Input: part model. Units: mm. Frame: model coordinates. A direction names the side the tool comes from. Coordinates: 2 decimals unless noted, no trailing zeros. Order: outer loops, then holes, each group sorted by start corner. A loop starts at its lowest first (then second) coordinate and runs counter-clockwise, first axis right, second up. Notation, with made-up numbers: M 50.25,-14 L 91.25,-14 A20 cw 91.25,17 Z; hole C 18.5,-23.75 d4. An arc over 180 degrees is marked long. Answer in a Markdown table with one row per item.
from build123d import *

# Parameters (mm, degrees)
ESQUISSE1_W             = 90
ESQUISSE1_H             = 65
ESQUISSE1_R             = 7
ESQUISSE1_R_2           = 13
BOSS_EXTRU_1_DEPTH      = 8
ESQUISSE2_R             = 13
BOSS_EXTRU_2_DEPTH      = 3
ESQUISSE3_R             = 7
ESQUISSE3_R_2           = 1.5
ENL_V_MAT_EXTRU_1_DEPTH = 4
ESQUISSE4_R             = 8
ENL_V_MAT_EXTRU_2_DEPTH = 5.5
ESQUISSE5_W             = 45
ESQUISSE5_H             = 8
ENL_V_MAT_EXTRU_3_DEPTH = 9
ESQUISSE6_R             = 1.65
ENL_V_MAT_EXTRU_4_DEPTH = 10
ESQUISSE7_R             = 1.65
ENL_V_MAT_EXTRU_5_DEPTH = 10


with BuildPart() as part:
    # Esquisse1 → Boss.-Extru.1 (new body)
    with BuildSketch(Plane.XY):
        with Locations((45, 32.5)):
            Rectangle(ESQUISSE1_W, ESQUISSE1_H)
        with Locations((70, 20)):
            Circle(ESQUISSE1_R, mode=Mode.SUBTRACT)
        with Locations((17, 20)):
            Circle(ESQUISSE1_R_2, mode=Mode.SUBTRACT)
        with Locations((25, 48)):
            Circle(ESQUISSE1_R_2, mode=Mode.SUBTRACT)
    extrude(amount=BOSS_EXTRU_1_DEPTH)

    # Esquisse2 → Boss.-Extru.2 (add)
    with BuildSketch(Plane(origin=(0, 0, 0), x_dir=(-1, 0, 0), z_dir=(0, 0, -1))):
        with Locations((-17, 20)):
            Circle(ESQUISSE2_R)
    extrude(amount=-BOSS_EXTRU_2_DEPTH)

    # Esquisse3 → Enlèv. mat.-Extru.1 (cut, through all)
    with BuildSketch(Plane.XY.offset(3)):
        with Locations((17, 20)):
            Circle(ESQUISSE3_R)
        with Locations((27, 20)):
            Circle(ESQUISSE3_R_2)
        with Locations((17, 10)):
            Circle(ESQUISSE3_R_2)
        with Locations((7, 20)):
            Circle(ESQUISSE3_R_2)
        with Locations((17, 30)):
            Circle(ESQUISSE3_R_2)
    extrude(amount=-ENL_V_MAT_EXTRU_1_DEPTH, mode=Mode.SUBTRACT)

    # Esquisse4 → Enlèv. mat.-Extru.2 (cut)
    with BuildSketch(Plane.XY.offset(8)):
        with Locations((70, 20)):
            Circle(ESQUISSE4_R)
    extrude(amount=-ENL_V_MAT_EXTRU_2_DEPTH, mode=Mode.SUBTRACT)

    # Esquisse5 → Enlèv. mat.-Extru.3 (cut, through all)
    with BuildSketch(Plane.XY.offset(8)):
        with Locations((67.5, 61)):
            Rectangle(ESQUISSE5_W, ESQUISSE5_H)
    extrude(amount=-ENL_V_MAT_EXTRU_3_DEPTH, mode=Mode.SUBTRACT)

    # Esquisse6 → Enlèv. mat.-Extru.4 (cut)
    with BuildSketch(Plane.ZY):
        with Locations((4, 7)):
            Circle(ESQUISSE6_R)
        with Locations((4, 45)):
            Circle(ESQUISSE6_R)
    extrude(amount=-ENL_V_MAT_EXTRU_4_DEPTH, mode=Mode.SUBTRACT)

    # Esquisse7 → Enlèv. mat.-Extru.5 (cut)
    with BuildSketch(Plane(origin=(0, 57, 0), x_dir=(1, 0, 0), z_dir=(0, 1, 0))):
        with Locations((85, -4)):
            Circle(ESQUISSE7_R)
        with Locations((55, -4)):
            Circle(ESQUISSE7_R)
    extrude(amount=-ENL_V_MAT_EXTRU_5_DEPTH, mode=Mode.SUBTRACT)


solid = part.part
1) Reachability of faces 1 (the face through (53.35, 52.07, 3.93)), 2 (the face through (10, 7, 4)), 3 (the face through (11, 14, 3)) from +Z, -Z, +X, -X, +Y, -Y: full face, straight path, thin tool, end or side. Return the list, or none.
Resolved:
| item | result |
|---|---|
| face 1 | +Y |
| face 2 | -X |
| face 3 | +Z |
2) Cut plane C-C, the plane x = 55. Output: boundary loops of the cut face in (y, z), and give its area (3 significant figures).
Resolved:
| item | result |
|---|---|
| outline | M 0,0 L 57,0 L 57,2.35 L 47,2.35 L 47,5.65 L 57,5.65 L 57,8 L 0,8 Z |
| area | 423 mm2 |
3) Cut plane B-B, the plane z = 4. Output: boundary loops of the cut face in (x, y), and give its area (3 significant figures).
Resolved:
| item | result |
|---|---|
| outline | M 0,0 L 90,0 L 90,57 L 86.65,57 L 86.65,47 L 83.35,47 L 83.35,57 L 56.65,57 L 56.65,47 L 53.35,47 L 53.35,57 L 45,57 L 45,65 L 0,65 L 0,46.65 L 10,46.65 L 10,43.35 L 0,43.35 L 0,8.65 L 10,8.65 L 10,5.35 L 0,5.35 Z; hole C 17,20 d26; hole C 25,48 d26; hole C 70,20 d16 |
| area | 4,100 mm2 |
4) Mould query, pull axis Y, two halves, no side actions, for faces 4 (the face through (22, 65, 4)), 5 (the face through (0, 32, 4)), 6 (the face through (44, 0, 4)), 7 (the face through (64.445, 15.741, 1.232)). Classes: +Y half, -Y half, draft (parallel to the pull), parting line (faces both ways), or undercut.
Resolved:
| item | result |
|---|---|
| face 4 | +Y half |
| face 5 | draft |
| face 6 | -Y half |
| face 7 | undercut |
5) Cut plane A-A, the plane y = 53. Output: boundary loops of the cut face in (x, z).
Resolved:
| item | result |
|---|---|
| outline | M 0,0 L 13,0 L 13,8 L 0,8 Z; M 37,0 L 90,0 L 90,8 L 37,8 Z; hole C 55,4 d3.3; hole C 85,4 d3.3 |
6) Material intervals for probe 1 along Z at (x, y) = (55, 55.25); probe 2 along X at (y, z) = (15, 1); probe 3 along Y at (x, z) = (27, 1.55), sorted ascending.
Resolved:
| item | result |
|---|---|
| probe 1 | z = 0 to 2.35, 5.65 to 8 |
| probe 2 | x = 0 to 12.1, 21.9 to 65.1, 74.9 to 90 |
| probe 3 | y = 0 to 18.5, 21.5 to 35.15, 60.85 to 65 |
7) Contact query for flat-ended pins moving along their axis: pin 1 (1.6 mm diameter, centred on x = 84, z = 4, fed in from +Y); pin 2 (13 mm diameter, centred on x = 21, y = 24, fed in from +Z); pin 3 (3.5 mm diameter, centred on x = 27, y = 20, fed in from -Z); pin 4 (3 mm diameter, centred on x = 55, z = 4, fed in from +Y). Output: stop coordinate, or through.
Resolved:
| item | result |
|---|---|
| pin 1 | stops at y = 57 |
| pin 2 | stops at z = 3 |
| pin 3 | stops at z = 0 |
| pin 4 | stops at y = 47 |
8) Cut plane D-D, the plane y = 20. Output: boundary loops of the cut face in (x, z).
Resolved:
| item | result |
|---|---|
| outline | M 0,0 L 5.5,0 L 5.5,3 L 4,3 L 4,8 L 0,8 Z; M 8.5,0 L 10,0 L 10,3 L 8.5,3 Z; M 24,0 L 25.5,0 L 25.5,3 L 24,3 Z; M 28.5,0 L 63,0 L 63,2.5 L 62,2.5 L 62,8 L 30,8 L 30,3 L 28.5,3 Z; M 77,0 L 90,0 L 90,8 L 78,8 L 78,2.5 L 77,2.5 Z |
